from build123d import *

# Parameters (mm, degrees)
BASE_FLANGE1_DEPTH   = 34
EDGE_FLANGE1_START   = -53.462169132
EDGE_FLANGE1_DEPTH   = 46.462169132
EDGE_FLANGE1_2_DEPTH = 46.462169132


# Read off the part's stored shape, not the designer's step: Edge-Flange1
# Sheet-metal steps are written as plain solids
with BuildPart() as part:
    # Sketch1 → Base-Flange1 (new body)
    with BuildSketch(Plane.XY):
        with BuildLine():
            Line((0, 0), (0, 56.743355504))
            ThreePointArc((0, 56.743355504), (-2.050252532, 61.693102972), (-7, 63.743355504))
            Line((-7, 63.743355504), (-53.462169132, 63.743355504))
            Line((-53.462169132, 63.743355504), (-53.462169132, 61.743355504))
            Line((-53.462169132, 61.743355504), (-7, 61.743355504))
            ThreePointArc((-7, 61.743355504), (-3.464466094, 60.278889409), (-2, 56.743355504))
            Line((-2, 56.743355504), (-2, 0))
            Line((-2, 0), (0, 0))
        make_face()
    extrude(amount=BASE_FLANGE1_DEPTH)

    # Edge-Flange1 outline → Edge-Flange1 (cut)
    with BuildSketch(Plane.YZ.offset(EDGE_FLANGE1_START)):
        with BuildLine():
            ThreePointArc((61.743355504, 29.958548116), (62.072211206, 32.078886242), (63.027879437, 34))
            Line((63.027879437, 34), (61.743355504, 34))
            Line((61.743355504, 34), (61.743355504, 29.958548116))
        make_face()
    extrude(amount=EDGE_FLANGE1_DEPTH, mode=Mode.SUBTRACT)

    # Edge-Flange1 2 outline → Edge-Flange1 2 (add)
    with BuildSketch(Plane.YZ.offset(EDGE_FLANGE1_START)):
        with BuildLine():
            Line((83.393990598, 46.5), (65.243355504, 36.020725942))
            ThreePointArc((65.243355504, 36.020725942), (64.026144133, 35.130386946), (63.027879437, 34))
            Line((63.027879437, 34), (63.743355504, 34))
            Line((63.743355504, 34), (63.743355504, 29.958548116))
            ThreePointArc((63.743355504, 29.958548116), (64.413228485, 32.458548116), (66.243355504, 34.288675135))
            Line((66.243355504, 34.288675135), (84.393990598, 44.767949192))
            Line((84.393990598, 44.767949192), (83.393990598, 46.5))
        make_face()
    extrude(amount=EDGE_FLANGE1_2_DEPTH)


solid = part.part
The model under review builds one solid part; all positions refer to its coordinate system, in mm. A direction names the side the tool comes from. Give positions to 0.01 mm unless a question says otherwise; leave off trailing zeros. Write each loop counter-clockwise with the first axis right and the second up, starting at its lowest first coordinate (ties: lowest second). Pieces come first, ordered by that corner, then holes. Notation, with made-up numbers: M -5,68.25 L 5,68.25 A23 cw 5,76.25 Z; hole C 2.5,19.5 d6. An arc over 180 degrees is marked long. One line per question, with ' | ' between items. Start each with the question number.
Item 1: We need section C-C on y = 12.5. Write out the cut boundary in (x, z), plus the area to 3 significant figures.
Item 2: For faces 1 (the flat face through (-53.462, 63, 27)), 2 (the flat face through (-2, 29, 17)), 3 (the flat face through (-30, 63.743, 15)), list the 3-axis set-ups (+Z, -Z, +X, -X, +Y, -Y) from which the entire face can be reached by the end or side of a thin tool; tool diameter is ignored.
Item 3: For pin 1 (1 mm diameter, centred on x = -22.5, y = 69.5, fed in from +Z); pin 2 (8 mm diameter, centred on x = -35, z = 31, fed in from -Y); pin 3 (10 mm diameter, centred on y = 54, z = 17.5, fed in from -X), all flat-tipped, find the tip position at first contact; note any pin that passes through.
Item 4: We need section A-A on z = 5. Write out the cut boundary in (x, y).
Item 5: We need section B-B on x = -42. Write out the cut boundary in (y, z).
Item 6: We need section D-D on y = 77. Write out the cut boundary in (x, z).
Item 7: Wall thickness on line 1 (X direction, y = 6.5, z = 4); line 2 (Y direction, x = -32, z = 10); line 3 (Y direction, x = -14, z = 36.5): over which ranges is each line inside the solid? List them lowest first. Write a range as from..to.
Results found:
1) outline: M -2,0 L 0,0 L 0,34 L -2,34 Z | area: 68.0 mm2
2) face 1: +Z, -Z, -X, +Y, -Y | face 2: +Z, -Z, -X, -Y | face 3: -Z, +X, -X, +Y
3) pin 1: stops at z = 38.77 | pin 2: stops at y = 61.74 | pin 3: stops at x = -2.54
4) outline: M -53.46,61.74 L -7,61.74 A5 cw -2,56.74 L -2,0 L 0,0 L 0,56.74 A7 ccw -7,63.74 L -53.46,63.74 Z
5) outline: M 61.74,0 L 63.74,0 L 63.74,29.96 A5 cw 66.24,34.29 L 84.39,44.77 L 83.39,46.5 L 65.24,36.02 A7 ccw 61.74,29.96 Z
6) outline: M -53.46,40.5 L -7,40.5 L -7,42.81 L -53.46,42.81 Z
7) line 1: x = -2..0 | line 2: y = 61.74..63.74 | line 3: y = 66.07..70.07
